Check sheet for the drawn part. Datum: minimum x, y, z corner. Units: mm. A direction names the side the tool comes from. Coordinates: 2 decimals unless noted, no trailing zeros. Write each loop counter-clockwise with the first axis right and the second up, starting at its lowest first coordinate (ties: lowest second). Pieces come first, ordered by that corner, then holes. Notation, with made-up numbers: (-9.75, 18) - (33.25, 18) arc R16 cw to (33.25, 32) - close; hole circle Ø6 at (-9, 3). An arc over 180 degrees is marked (long way). Write each question's results on one line, items separated by ' | '.
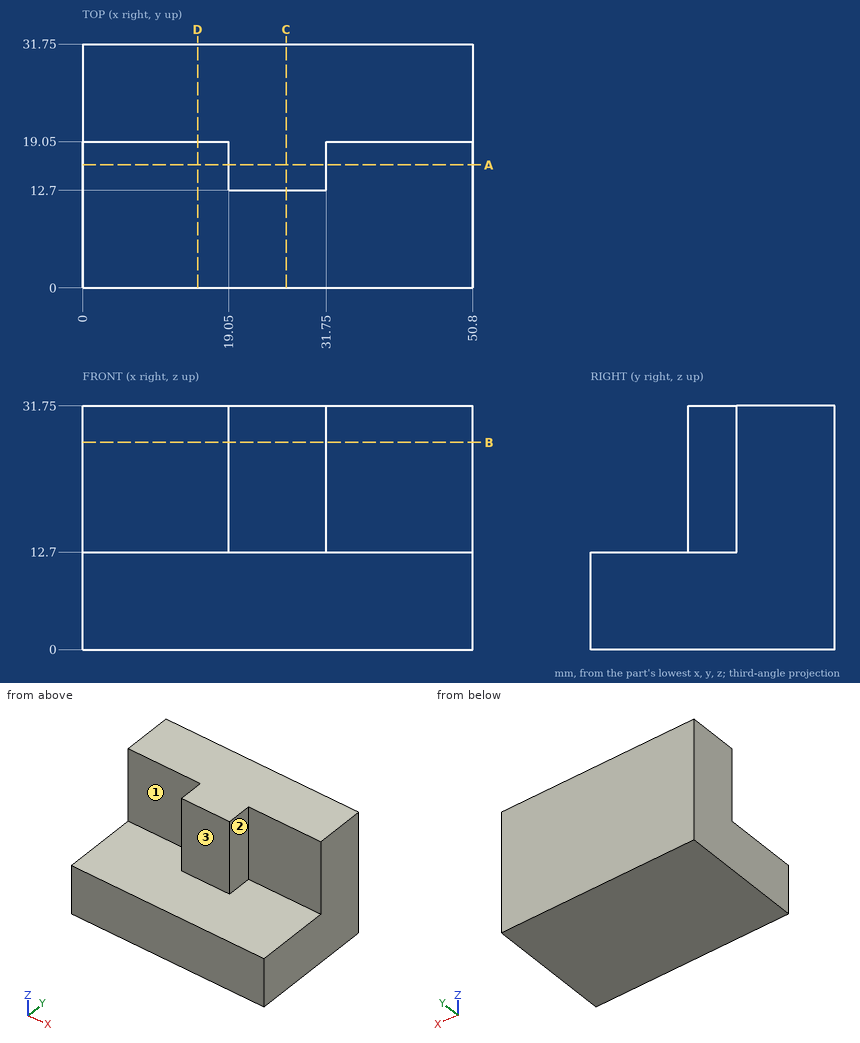
1. Sectioned sample at D-D (x = 15). Record the cut outline in (y, z), then the cut area to 3 significant figures.
Values follow:
outline: (0, 0) - (31.75, 0) - (31.75, 31.75) - (19.05, 31.75) - (19.05, 12.7) - (0, 12.7) - close | area: 645 mm^2
2. Go/stop test with flat-tipped pins: pin 1 (1.9 mm diameter, centred on y = 15, z = 25.5, fed in from +X); pin 2 (3 mm diameter, centred on y = 14.5, z = 25.5, fed in from -X); pin 3 (10 mm diameter, centred on x = 27.5, z = 24, fed in from -Y). Record where each tip stops, or that it passes through.
Values follow:
pin 1: stops at x = 31.75 | pin 2: stops at x = 19.05 | pin 3: stops at y = 12.7
3. Sectioned sample at C-C (x = 26.5). Record the cut outline in (y, z), then the cut area to 3 significant figures.
Values follow:
outline: (0, 0) - (31.75, 0) - (31.75, 31.75) - (12.7, 31.75) - (12.7, 12.7) - (0, 12.7) - close | area: 766 mm^2
4. Sectioned sample at A-A (y = 16). Record the cut outline in (x, z).
Values follow:
outline: (0, 0) - (50.8, 0) - (50.8, 12.7) - (31.75, 12.7) - (31.75, 31.75) - (19.05, 31.75) - (19.05, 12.7) - (0, 12.7) - close
5. Material ranges on L1, parallel to Z at x = 22.5, y = 4; L2, parallel to Y at x = 45, z = 26; L3, parallel to Y at x = 29, z = 21.5, recorded low to high. Write a range as [from, to].
Values follow:
L1: z = [0, 12.7] | L2: y = [19.05, 31.75] | L3: y = [12.7, 31.75]
6. Sectioned sample at B-B (z = 27). Record the cut outline in (x, y), then the cut area to 3 significant figures.
Values follow:
outline: (0, 19.05) - (19.05, 19.05) - (19.05, 12.7) - (31.75, 12.7) - (31.75, 19.05) - (50.8, 19.05) - (50.8, 31.75) - (0, 31.75) - close | area: 726 mm^2
7. Access from +Z, -Z, +X, -X, +Y, -Y to the whole of each face (thin tool, end or side, straight path). Record for the marked faces 1, 2 and 3.
Values follow:
face 1: +Z, -X, -Y | face 2: +Z, +X, -Y | face 3: +Z, +X, -X, -Y
